Check sheet for the drawn part. Datum: minimum x, y, z corner. Units: mm. A direction names the side the tool comes from. Give positions to 0.01 mm unless a question says otherwise; leave off trailing zeros. Order: outer loops, then holes, each group sorted by start corner. A loop starts at its lowest first (then second) coordinate and runs counter-clockwise, first axis right, second up. Notation, with made-up numbers: M -35,52 L 10,52 A12 ccw 10,67 Z; hole C 29.25,66 d8. An arc over 180 degrees is marked long. Put each result on its own line as item: value. Start each with the question number.
Q1. Section check D-D on z = 42. Record the cut outline in (x, y).
Q2. Section check A-A on x = 43.5. Record the cut outline in (y, z), then the cut area to 3 significant figures.
Q3. Section check B-B on z = 21.5. Record the cut outline in (x, y), then the cut area to 3 significant figures.
Q4. Go/stop test with flat-tipped pins: pin 1 (11 mm diameter, centred on y = 12, z = 18, fed in from -X); pin 2 (5.5 mm diameter, centred on x = 51, y = 6, fed in from +Z); pin 3 (8 mm diameter, centred on x = 37.5, y = 13.5, fed in from +Z); pin 4 (8 mm diameter, centred on x = 53, z = 27.5, fed in from +Y). Record where each tip stops, or that it passes through.
Q5. Section check C-C on y = 15. Record the cut outline in (x, z).
Q6. Access from +Z, -Z, +X, -X, +Y, -Y to the whole of each face (thin tool, end or side, straight path). Record for the marked faces 1 and 2.
Q7. Material ranges on L1, parallel to X at y = 6.5, z = 9; L2, parallel to X at y = 9, z = 46; L3, parallel to Y at x = 67, z = 39.5, recorded low to high.
Q8. Mould release check, pull along X, two halves, no side actions. Record for the marked faces 3, 4, 5 and 6: +X half, -X half, draft (parallel to the pull), parting line (faces both ways), or undercut.
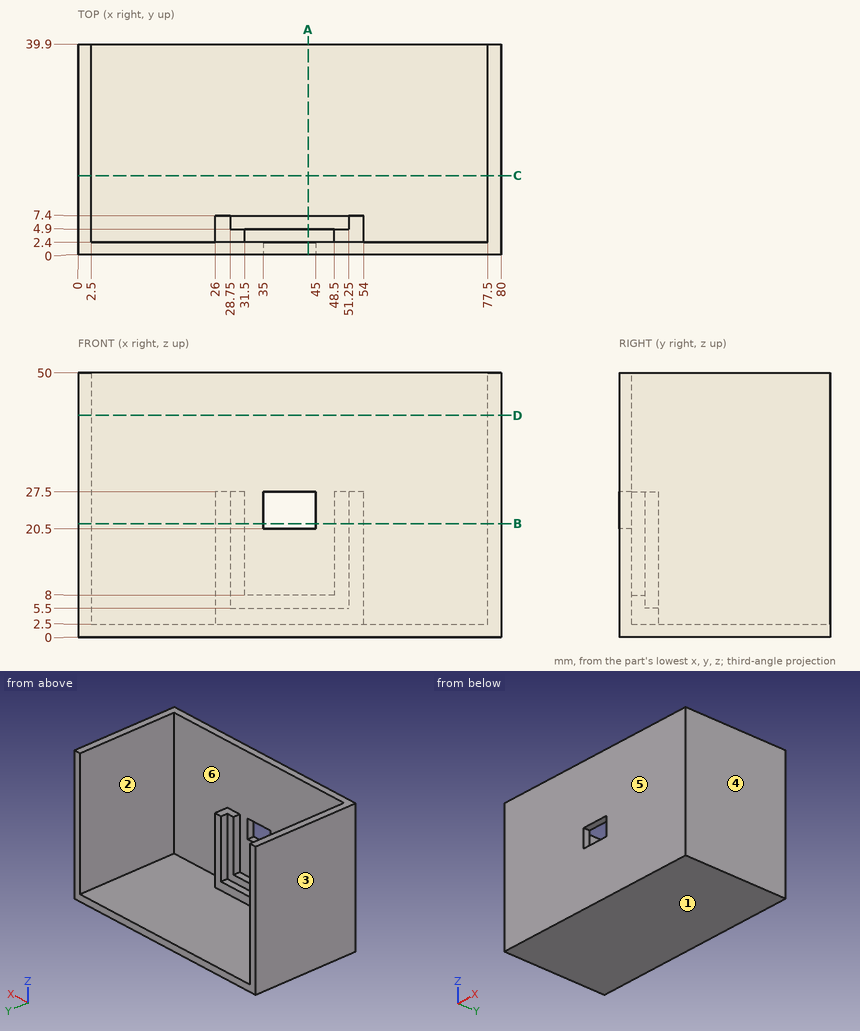
Results found:
1. outline: M 0,0 L 80,0 L 80,39.9 L 77.5,39.9 L 77.5,2.4 L 2.5,2.4 L 2.5,39.9 L 0,39.9 Z
2. outline: M 0,0 L 39.9,0 L 39.9,2.5 L 7.4,2.5 L 7.4,5.5 L 4.9,5.5 L 4.9,8 L 2.4,8 L 2.4,20.5 L 0,20.5 Z; M 0,27.5 L 2.4,27.5 L 2.4,50 L 0,50 Z
2. area: 218 mm^2
3. outline: M 0,0 L 35,0 L 35,2.4 L 31.5,2.4 L 31.5,4.9 L 28.75,4.9 L 28.75,7.4 L 26,7.4 L 26,2.4 L 2.5,2.4 L 2.5,39.9 L 0,39.9 Z; M 45,0 L 80,0 L 80,39.9 L 77.5,39.9 L 77.5,2.4 L 54,2.4 L 54,7.4 L 51.25,7.4 L 51.25,4.9 L 48.5,4.9 L 48.5,2.4 L 45,2.4 Z
3. area: 397 mm^2
4. pin 1: stops at x = 0
4. pin 2: stops at z = 27.5
4. pin 3: stops at z = 2.5
4. pin 4: stops at y = 7.4
5. outline: M 0,0 L 80,0 L 80,50 L 77.5,50 L 77.5,2.5 L 2.5,2.5 L 2.5,50 L 0,50 Z
6. face 1: -Z, +X, -X, +Y, -Y
6. face 2: +Z, +Y
7. L1: x = 0 to 2.5, 26 to 28.75, 51.25 to 54, 77.5 to 80
7. L2: x = 0 to 2.5, 77.5 to 80
7. L3: y = 0 to 2.4
8. face 3: -X half
8. face 4: +X half
8. face 5: draft
8. face 6: undercut
